Can you work these out from the model? Positions are in its coordinate system, mm. A direction names the side the tool comes from. Round coordinates to 2 decimals unless told otherwise and drop trailing zeros. Order: outer loops, then holes, each group sorted by start corner. A loop starts at its lowest first (then second) coordinate and runs counter-clockwise, first axis right, second up.
Q1. If we section it at A-A (z = 6.5): Please give me the cut outline in (x, y).
Q2. For faces 1 (the face through (0, 2.25, 1)), 2 (the face through (16.25, 0, 6)), 3 (the face through (14.75, 0, 12)), which set-ups out of +Z, -Z, +X, -X, +Y, -Y let a thin tool reach every point of the face, with its end or its side?
Q3. If I drill on line 1 (X direction, y = 3.25, z = 12.5); line 2 (X direction, y = -1.25, z = 4.5); line 3 (Z direction, x = 1, y = 2), over which ranges is the centre line in solid material (lowest first)?
Q4. If we section it at C-C (x = 5.5): Please give me the cut outline in (y, z).
Q5. Will these pins go through, and if not, where does the flat tip stop? P1, Ø2, axis at x = 1, y = 1, coming from the -Z side (3 decimals); P2, Ø6, axis at x = -5.5, z = -3.5, coming from the -Y side; P3, Ø5, axis at y = 2.5, z = -5, coming from the -X side; P4, Ø5, axis at x = 1, z = 7.5, coming from the -Y side.
Q6. We'd pull the mould along X, two halves only. Please class faces 4 (the face through (-16, -4.521, 14)), 5 (the face through (-17.65, 0, 14)), 6 (the face through (-1.43, -0.45, 2.49)): pulls with the +X half, pulls with the -X half, needs draft (parallel to the pull), parting line crosses it, or undercut.
Q7. If we section it at D-D (x = -3): Please give me the cut outline in (y, z), plus the area to 3 significant figures.
from build123d import *

# Parameters (mm, degrees)
EXTRUDE_2_DEPTH        = 2.25
EXTRUDE_4_DEPTH        = 0.9
EXTRUDE_5_DEPTH        = 2.9
FILLET_1_R             = 1.2
FILLET_1_OF_MIRROR_2_R = 1.2
SKETCH_3_R             = 1.5
EXTRUDE_6_DEPTH        = 2


with BuildPart() as part:
    # Sketch 1 → Extrude 2 (new, symmetric)
    with BuildSketch(Plane(origin=(0, 0, 0), x_dir=(1, 0, 0), z_dir=(0, 1, 0))):
        with BuildLine():
            Line((-12.75, -1.5), (12.75, -1.5))
            ThreePointArc((12.75, -1.5), (14.164213562, -2.085786438), (14.75, -3.5))
            Line((14.75, -3.5), (14.75, -9.3))
            Line((14.75, -9.3), (16.25, -9.3))
            Line((16.25, -9.3), (16.25, -3.5))
            ThreePointArc((16.25, -3.5), (15.224873734, -1.025126266), (12.75, 0))
            Line((12.75, 0), (-12.75, 0))
            ThreePointArc((-12.75, 0), (-15.224873734, -1.025126266), (-16.25, -3.5))
            Line((-16.25, -3.5), (-16.25, -9.3))
            Line((-16.25, -9.3), (-14.75, -9.3))
            Line((-14.75, -9.3), (-14.75, -3.5))
            ThreePointArc((-14.75, -3.5), (-14.164213562, -2.085786438), (-12.75, -1.5))
        make_face()
    extrude(amount=EXTRUDE_2_DEPTH, both=True)

    # Sketch 1_6 → Extrude 4 (add, symmetric)
    with BuildSketch(Plane(origin=(0, 0, 0), x_dir=(1, 0, 0), z_dir=(0, 1, 0))):
        Polygon((9.278174593, 7.778174593), (1.5, 0), (4.045584412, 0), (10.550966799, 6.505382387), align=None)
        Polygon((-4.045584412, 0), (-1.5, 0), (-9.278174593, 7.778174593), (-10.550966799, 6.505382387), align=None)
    extrude(amount=EXTRUDE_4_DEPTH, both=True)

    # Sketch 2 → Extrude 5 (add)
    with BuildSketch(Plane.ZY.offset(-14.75)):
        with BuildLine():
            Line((16.3, 4.478921871), (11.3, 4.478921871))
            ThreePointArc((11.3, 4.478921871), (9.885786438, 3.893135433), (9.3, 2.478921871))
            Line((9.3, 2.478921871), (9.3, -2.521078129))
            ThreePointArc((9.3, -2.521078129), (9.885786438, -3.935291691), (11.3, -4.521078129))
            Line((11.3, -4.521078129), (16.3, -4.521078129))
            ThreePointArc((16.3, -4.521078129), (17.714213562, -3.935291691), (18.3, -2.521078129))
            Line((18.3, -2.521078129), (18.3, 2.478921871))
            ThreePointArc((18.3, 2.478921871), (17.714213562, 3.893135433), (16.3, 4.478921871))
        make_face()
    extrude_5 = extrude(amount=-EXTRUDE_5_DEPTH)

    # Fillet 1
    fillet_1_edges = [part.edges().sort_by_distance(p)[0] for p in [
        (17.65, 3.893135433, 9.885786438),
        (17.65, 4.478921871, 13.8),
        (17.65, 3.893135433, 17.714213562),
        (17.65, -0.021078129, 18.3),
        (17.65, -3.935291691, 17.714213562),
        (17.65, -4.521078129, 13.8),
        (17.65, -3.935291691, 9.885786438),
        (17.65, -0.021078129, 9.3),
    ]]
    fillet(fillet_1_edges, radius=FILLET_1_R)

    # Mirror 2: Extrude 5 across plane
    add(extrude_5.mirror(Plane(origin=(0, 0, 0), x_dir=(0, 0, 1), z_dir=(1, 0, 0))))

    # Fillet 1 of Mirror 2
    fillet_1_of_mirror_2_edges = [part.edges().sort_by_distance(p)[0] for p in [
        (-17.65, 3.893135433, 9.885786438),
        (-17.65, 4.478921871, 13.8),
        (-17.65, 3.893135433, 17.714213562),
        (-17.65, -0.021078129, 18.3),
        (-17.65, -3.935291691, 17.714213562),
        (-17.65, -4.521078129, 13.8),
        (-17.65, -3.935291691, 9.885786438),
        (-17.65, -0.021078129, 9.3),
    ]]
    fillet(fillet_1_of_mirror_2_edges, radius=FILLET_1_OF_MIRROR_2_R)

    # Sketch 3 → Extrude 6 (add)
    with BuildSketch(Plane.XY.offset(1.5)):
        with Locations(Location((0, 0, 0), (0, 0, 180))):
            Circle(SKETCH_3_R)
    extrude(amount=EXTRUDE_6_DEPTH)


solid = part.part
Solution:
1. outline: (-16.25, -2.25) - (-14.75, -2.25) - (-14.75, 2.25) - (-16.25, 2.25) - close; (14.75, -2.25) - (16.25, -2.25) - (16.25, 2.25) - (14.75, 2.25) - close
2. face 1: -Z, +X, -X, +Y
2. face 2: -Z, +X, +Y, -Y
2. face 3: +Z, +Y, -Y
3. line 1: x = -17.65 to -14.75, 14.75 to 17.65
3. line 2: x = -16.25 to -14.75, 14.75 to 16.25
3. line 3: z = 0 to 1.5
4. outline: (-2.25, 0) - (2.25, 0) - (2.25, 1.5) - (-2.25, 1.5) - close; (-0.9, -4) - (0.9, -4) - (0.9, -1.45) - (-0.9, -1.45) - close
5. P1: stops at z = -0.495
5. P2: stops at y = -0.9
5. P3: stops at x = -10.55
5. P4: passes through
6. face 4: needs draft
6. face 5: pulls with the -X half
6. face 6: undercut
7. outline: (-2.25, 0) - (-0.9, 0) - (-0.9, -1.5) - (0.9, -1.5) - (0.9, 0) - (2.25, 0) - (2.25, 1.5) - (-2.25, 1.5) - close
7. area: 9.45 mm2
